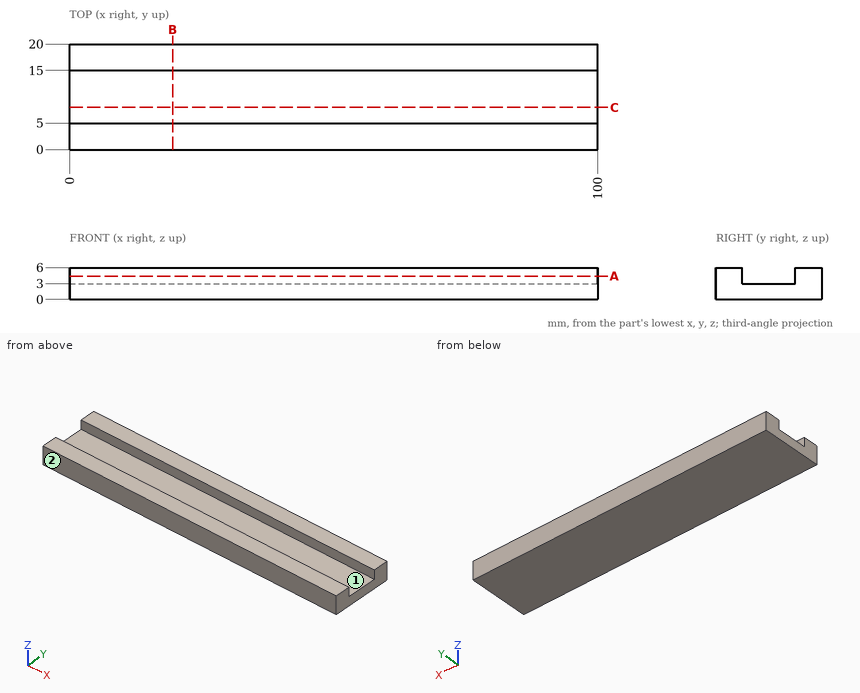
Design review of the part shown in the three views and the two pictorial views. Dimensions are in mm from the part's minimum x, y and z. A direction names the side the tool comes from. Coordinates: 2 decimals unless noted, no trailing zeros. Order: outer loops, then holes, each group sorted by start corner. A loop starts at its lowest first (then second) coordinate and runs counter-clockwise, first axis right, second up.
1) Wall thickness on line 1 along Y through (x, z) = (5.5, 4.05); line 2 along Z through (x, y) = (70.5, 8.25): over which ranges is each line inside the solid? List them lowest first.
2) Take a section at A-A, the plane z = 4.4. Give the boundary of the cut face in (x, y).
3) Take a section at C-C, the plane y = 8. Give the boundary of the cut face in (x, z), and give its area (3 significant figures).
4) Take a section at B-B, the plane x = 19.5. Give the boundary of the cut face in (y, z), and give its area (3 significant figures).
5) For the marked faces 1 and 2, list the 3-axis set-ups (+Z, -Z, +X, -X, +Y, -Y) from which the entire face can be reached by the end or side of a thin tool; tool diameter is ignored.
Returned:
1. line 1: y = 0 to 5, 15 to 20
1. line 2: z = 0 to 3
2. outline: (0, 0) - (100, 0) - (100, 5) - (0, 5) - close; (0, 15) - (100, 15) - (100, 20) - (0, 20) - close
3. outline: (0, 0) - (100, 0) - (100, 3) - (0, 3) - close
3. area: 300 mm2
4. outline: (0, 0) - (20, 0) - (20, 6) - (15, 6) - (15, 3) - (5, 3) - (5, 6) - (0, 6) - close
4. area: 90.0 mm2
5. face 1: +Z, +X, -X
5. face 2: +Z, -Z, +X, -X, -Y
